Job drawing, mm, ordinate dimensions from the low corner. One solid piece. A direction names the side the tool comes from. Give positions to 0.01 mm unless a question says otherwise; leave off trailing zeros. Write each loop counter-clockwise with the first axis right and the second up, starting at its lowest first coordinate (ties: lowest second). Pieces come first, ordered by that corner, then holes. Notation, with made-up numbers: (-11, 0.25) -> (42, 0.25) arc R27 cw to (42, 18.25) -> close; hole circle Ø3 at (25.5, 80.25). An arc over 180 degrees is marked (long way). One line per question, with ' | ' between items. Start each with the question number.
(1) Band-saw the part on D-D, the plane x = 7. Give the cut face in (y, z).
(2) Pin check, flat tips, straight feed: P1, Ø1.8, axis at x = 27.125, z = 8, coming from the +Y side (3 decimals); P2, Ø5, axis at y = 7, z = 13.5, coming from the +X side; P3, Ø5, axis at x = 6, z = 2, coming from the -Y side; P4, Ø4.5, axis at x = 29, z = 10, coming from the -Y side. Stop position of each tip, or through.
(3) Tool access for the marked faces 5, 6 and 7: list every direction of +Z, -Z, +X, -X, +Y, -Y with a clear straight run to the whole face (end or side of a thin tool).
(4) Band-saw the part on A-A, the plane z = 6.25. Give the cut face in (x, y).
(5) Pull direction Z, two halves, no side cores. Call the marked faces 1, 2, 3 and 4: released by +Z, released by -Z, zero draft, split by the parting line, or undercut.
(6) Band-saw the part on C-C, the plane z = 8. Give the cut face in (x, y) (3 decimals), and give its area (4 significant figures).
(7) Drill centre lines: probe 1 along Z at (x, y) = (13.5, 2.5); probe 2 along X at (y, z) = (15.45, 8) (3 decimals); probe 3 along X at (y, z) = (7, 13.75). Where is each one in solid material? Low to high. Write a range as from..to.
(8) Band-saw the part on B-B, the plane y = 8. Give the cut face in (x, z), and give its area (3 significant figures).
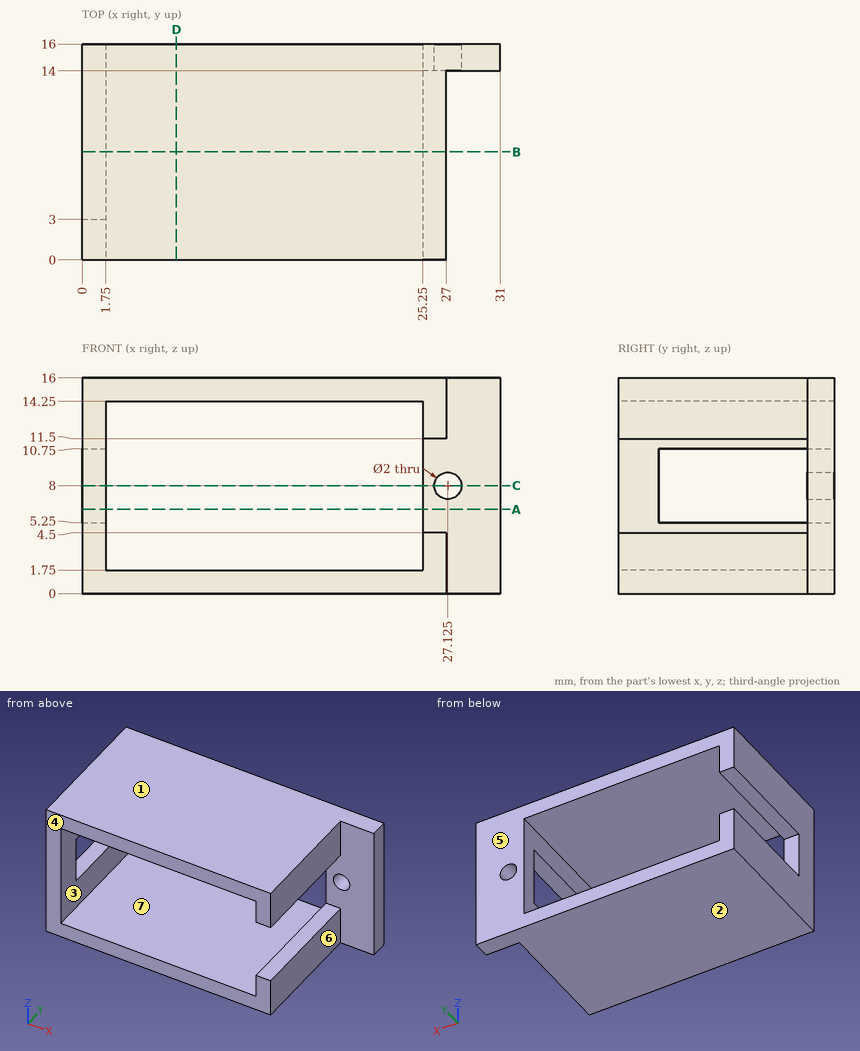
Results:
1) outline: (0, 0) -> (16, 0) -> (16, 1.75) -> (0, 1.75) -> close; (0, 14.25) -> (16, 14.25) -> (16, 16) -> (0, 16) -> close
2) P1: passes through | P2: stops at x = 27 | P3: stops at y = 0 | P4: stops at y = 14
3) face 5: +Z, -Z, +X, -X, +Y | face 6: +Z, -Z, +X, -Y | face 7: +Y, -Y
4) outline: (0, 0) -> (1.75, 0) -> (1.75, 3) -> (0, 3) -> close; (25.25, 14) -> (31, 14) -> (31, 16) -> (25.25, 16) -> close
5) face 1: released by +Z | face 2: released by -Z | face 3: undercut | face 4: zero draft
6) outline: (0, 0) -> (1.75, 0) -> (1.75, 3) -> (0, 3) -> close; (25.25, 14) -> (26.125, 14) -> (26.125, 16) -> (25.25, 16) -> close; (28.125, 14) -> (31, 14) -> (31, 16) -> (28.125, 16) -> close | area: 12.75 mm²
7) probe 1: z = 0..1.75, 14.25..16 | probe 2: x = 25.25..26.125, 28.125..31 | probe 3: x = 0..1.75, 25.25..27
8) outline: (0, 0) -> (27, 0) -> (27, 4.5) -> (25.25, 4.5) -> (25.25, 1.75) -> (1.75, 1.75) -> (1.75, 5.25) -> (0, 5.25) -> close; (0, 10.75) -> (1.75, 10.75) -> (1.75, 14.25) -> (25.25, 14.25) -> (25.25, 11.5) -> (27, 11.5) -> (27, 16) -> (0, 16) -> close | area: 116 mm²
